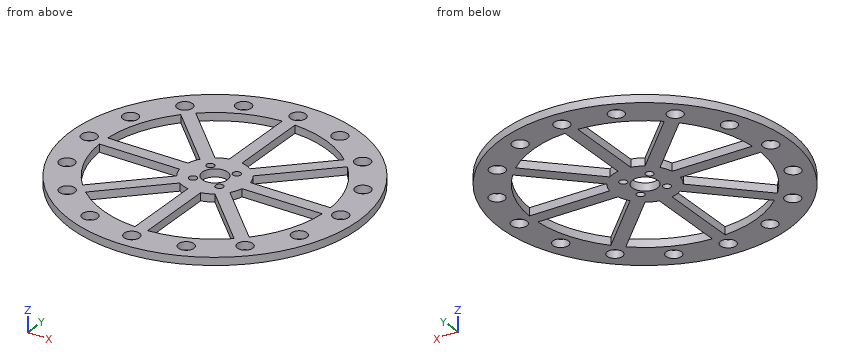
```python
from build123d import *

# Parameters (mm, degrees)
MODEL_R             = 58.667489702
MODEL_R_2           = 1.591156764
MODEL_R_3           = 5.125
MODEL_R_4           = 3.130979628
BOSS_EXTRUDE1_DEPTH = 3.175


with BuildPart() as part:
    # Model → Boss-Extrude1 (new body)
    with BuildSketch(Plane.XY):
        Circle(MODEL_R)
        with Locations((5.389401941, 5.35857693)):
            Circle(MODEL_R_2, mode=Mode.SUBTRACT)
        Circle(MODEL_R_3, mode=Mode.SUBTRACT)
        with Locations((-5.389401941, 5.35857693)):
            Circle(MODEL_R_2, mode=Mode.SUBTRACT)
        with Locations((-5.389401941, -5.420226952)):
            Circle(MODEL_R_2, mode=Mode.SUBTRACT)
        with Locations((5.389401941, -5.420226952)):
            Circle(MODEL_R_2, mode=Mode.SUBTRACT)
        with Locations((-51.409488894, 0)):
            Circle(MODEL_R_4, mode=Mode.SUBTRACT)
        with Locations((-47.496174566, 19.673559666)):
            Circle(MODEL_R_4, mode=Mode.SUBTRACT)
        with Locations((-36.351998214, 36.351998214)):
            Circle(MODEL_R_4, mode=Mode.SUBTRACT)
        with Locations((-19.673559666, 47.496174566)):
            Circle(MODEL_R_4, mode=Mode.SUBTRACT)
        with Locations((0, 51.409488894)):
            Circle(MODEL_R_4, mode=Mode.SUBTRACT)
        with Locations((19.673559666, 47.496174566)):
            Circle(MODEL_R_4, mode=Mode.SUBTRACT)
        with Locations((36.351998214, 36.351998214)):
            Circle(MODEL_R_4, mode=Mode.SUBTRACT)
        with Locations((47.496174566, 19.673559666)):
            Circle(MODEL_R_4, mode=Mode.SUBTRACT)
        with Locations((51.409488894, 0)):
            Circle(MODEL_R_4, mode=Mode.SUBTRACT)
        with Locations((47.496174566, -19.673559666)):
            Circle(MODEL_R_4, mode=Mode.SUBTRACT)
        with Locations((36.351998214, -36.351998214)):
            Circle(MODEL_R_4, mode=Mode.SUBTRACT)
        with Locations((19.673559666, -47.496174566)):
            Circle(MODEL_R_4, mode=Mode.SUBTRACT)
        with Locations((0, -51.409488894)):
            Circle(MODEL_R_4, mode=Mode.SUBTRACT)
        with Locations((-19.673559666, -47.496174566)):
            Circle(MODEL_R_4, mode=Mode.SUBTRACT)
        with Locations((-36.351998214, -36.351998214)):
            Circle(MODEL_R_4, mode=Mode.SUBTRACT)
        with Locations((-47.496174566, -19.673559666)):
            Circle(MODEL_R_4, mode=Mode.SUBTRACT)
        with BuildLine():
            Line((-34.056493108, 30.369010459), (-10.87619225, 7.188709601))
            ThreePointArc((-10.87619225, 7.188709601), (-12.044820658, 4.989128073), (-12.773814601, 2.607443987))
            Line((-12.773814601, 2.607443987), (-45.555710454, 2.607443987))
            ThreePointArc((-45.555710454, 2.607443987), (-42.156872302, 17.461948255), (-34.056493108, 30.369010459))
        make_face(mode=Mode.SUBTRACT)
        with BuildLine():
            Line((-7.188709601, 10.87619225), (-30.369010459, 34.056493108))
            ThreePointArc((-30.369010459, 34.056493108), (-17.461948255, 42.156872302), (-2.607443987, 45.555710454))
            Line((-2.607443987, 45.555710454), (-2.607443987, 12.773814601))
            ThreePointArc((-2.607443987, 12.773814601), (-4.989128073, 12.044820658), (-7.188709601, 10.87619225))
        make_face(mode=Mode.SUBTRACT)
        with BuildLine():
            Line((2.607443987, 12.773814601), (2.607443987, 45.555710454))
            ThreePointArc((2.607443987, 45.555710454), (17.461948254, 42.156872302), (30.369010459, 34.056493108))
            Line((30.369010459, 34.056493108), (7.188709601, 10.87619225))
            ThreePointArc((7.188709601, 10.87619225), (4.989128073, 12.044820658), (2.607443987, 12.773814601))
        make_face(mode=Mode.SUBTRACT)
        with BuildLine():
            Line((10.87619225, 7.188709601), (34.056493108, 30.369010459))
            ThreePointArc((34.056493108, 30.369010459), (42.156872302, 17.461948255), (45.555710454, 2.607443987))
            Line((45.555710454, 2.607443987), (12.773814601, 2.607443987))
            ThreePointArc((12.773814601, 2.607443987), (12.044820658, 4.989128073), (10.87619225, 7.188709601))
        make_face(mode=Mode.SUBTRACT)
        with BuildLine():
            Line((12.773814601, -2.607443987), (45.555710454, -2.607443987))
            ThreePointArc((45.555710454, -2.607443987), (42.156872302, -17.461948254), (34.056493108, -30.369010459))
            Line((34.056493108, -30.369010459), (10.87619225, -7.188709601))
            ThreePointArc((10.87619225, -7.188709601), (12.044820658, -4.989128073), (12.773814601, -2.607443987))
        make_face(mode=Mode.SUBTRACT)
        with BuildLine():
            Line((7.188709601, -10.87619225), (30.369010459, -34.056493108))
            ThreePointArc((30.369010459, -34.056493108), (17.461948255, -42.156872302), (2.607443987, -45.555710454))
            Line((2.607443987, -45.555710454), (2.607443987, -12.773814601))
            ThreePointArc((2.607443987, -12.773814601), (4.989128073, -12.044820658), (7.188709601, -10.87619225))
        make_face(mode=Mode.SUBTRACT)
        with BuildLine():
            Line((-45.555710454, -2.607443987), (-12.773814601, -2.607443987))
            ThreePointArc((-12.773814601, -2.607443987), (-12.044820658, -4.989128073), (-10.87619225, -7.188709601))
            Line((-10.87619225, -7.188709601), (-34.056493108, -30.369010459))
            ThreePointArc((-34.056493108, -30.369010459), (-42.156872302, -17.461948254), (-45.555710454, -2.607443987))
        make_face(mode=Mode.SUBTRACT)
        with BuildLine():
            Line((-2.607443987, -12.773814601), (-2.607443987, -45.555710454))
            ThreePointArc((-2.607443987, -45.555710454), (-17.461948255, -42.156872302), (-30.369010459, -34.056493108))
            Line((-30.369010459, -34.056493108), (-7.188709601, -10.87619225))
            ThreePointArc((-7.188709601, -10.87619225), (-4.989128073, -12.044820658), (-2.607443987, -12.773814601))
        make_face(mode=Mode.SUBTRACT)
    extrude(amount=BOSS_EXTRUDE1_DEPTH)


solid = part.part
```
Geometry check sheet. Reference: the model listing, model coordinates, mm. Give positions to 0.01 mm unless a question says otherwise; leave off trailing zeros. Order: outer loops, then holes, each group sorted by start corner. A loop starts at its lowest first (then second) coordinate and runs counter-clockwise, first axis right, second up.
1. Thickness scan on L1, parallel to Y at x = 0, z = 0.9 (1 decimal); L2, parallel to Y at x = -4, z = 1.2; L3, parallel to Y at x = -6.5, z = 2.4. Record the ranges inside material, lowest first.
2. Gauge pin test, flat ends, axial feed: pin 1 Ø1 at (x, z) = (42.5, 2) entering from -Y; pin 2 Ø1.5 at (y, z) = (45, 2.5) entering from -X; pin 3 Ø1 at (x, z) = (27.5, 1.5) entering from +Y. Record the tip position at first contact, or that the pin passes through.
3. Section check C-C, the plane z = 1.25. Give the number of separate pieces and of enclosed holes in the cut face, and give its area (3 significant figures).
4. Section check A-A, the plane x = 0. Enter the section's corners in (y, z) (1 decimal).
Values follow:
1. L1: y = -58.7 to -54.5, -48.3 to -5.1, 5.1 to 48.3, 54.5 to 58.7
1. L2: y = -58.53 to -45.45, -12.41 to -6.2, -4.64 to -3.2, 3.2 to 4.58, 6.13 to 12.41, 45.45 to 58.53
1. L3: y = -58.31 to -45.16, -11.3 to -6.56, -4.28 to 4.22, 6.5 to 11.3, 45.16 to 58.31
2. pin 1: stops at y = -40.96
2. pin 2: stops at x = -38.52
2. pin 3: stops at y = 52.09
3. separate pieces: 1
3. enclosed holes: 29
3. area: 5,560 mm2
4. outline: (-58.7, 0) - (-54.5, 0) - (-54.5, 3.2) - (-58.7, 3.2) - close; (-48.3, 0) - (-5.1, 0) - (-5.1, 3.2) - (-48.3, 3.2) - close; (5.1, 0) - (48.3, 0) - (48.3, 3.2) - (5.1, 3.2) - close; (54.5, 0) - (58.7, 0) - (58.7, 3.2) - (54.5, 3.2) - close
